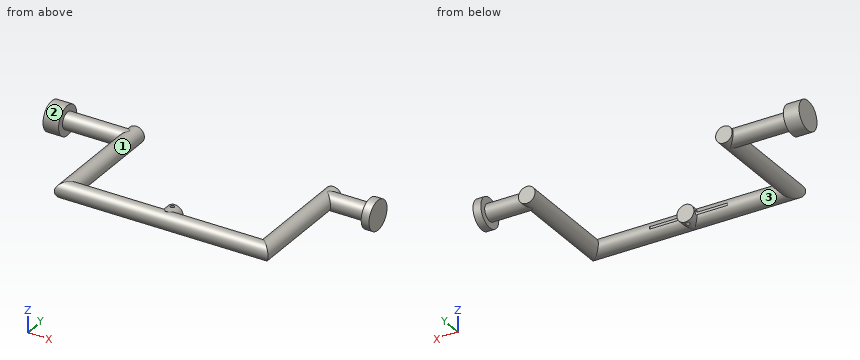
Autodesk Inventor part; units mm, degrees
ref_plane "Work Plane1" through (-126.3, 142.5, 0) normal (0, 1, 0) x (-1, 0, 0)
ref_plane "Work Plane2" through (0, 0, 0) normal (0, 1, 0) x (-1, 0, 0)
ref_plane "Work Plane3" through (0, 0, 0) normal (0, 0, 1) x (1, 0, 0)
sketch "Sketch1" plane through (0, 0, 0) normal (0, 0, 1) x (1, 0, 0)
  line L0 (-126.3, 0) -> (126.3, 0)
  line L1 (126.3, 0) -> (126.3, 142.5)
  line L2 (126.3, 0) -> (268.8, 0) construction
  line L3 (-126.3, 0) -> (-126.3, 142.5)
  point P0 (0, 0)
  dimension "d0" = 252.6
  dimension "d1" = 142.5
  dimension "d2" = 90
  dimension "d3" = 142.5
ref_plane "Work Plane1" through (-126.3, 142.5, 0) normal (0, 1, 0) x (-1, 0, 0)
sketch "Sketch2" plane through (-126.3, 142.5, 0) normal (0, 1, 0) x (-1, 0, 0)
  circle A0 centre (0, 0) radius 10.65
  point P0 (-126.3, 0)
  dimension "d4" = 21.3
sweep "Sweep1" add profiles "Sketch2" path "Sketch1"
ref_plane "Work Plane2" through (0, 0, 0) normal (0, 1, 0) x (-1, 0, 0)
sketch "Sketch3" plane through (0, 0, 0) normal (0, 1, 0) x (-1, 0, 0)
  circle A0 centre (0, 0) radius 11
  dimension "d8" = 22
extrude "Extrusion1" add sketch "Sketch3" along normal blind 17.5
ref_plane "Work Plane3" through (0, 0, 0) normal (0, 0, 1) x (1, 0, 0)
sketch "Sketch4" plane through (0, 0, 0) normal (0, 0, 1) x (1, 0, 0)
  circle A0 centre (0, 12.5) radius 2.5
  point P0 (0, 0)
  dimension "d12" = 5
extrude "Extrusion2" cut sketch "Sketch4" along normal mid plane 100
ref_plane "Work Plane4" through (0, 0, 0) normal (1, 0, 0) x (0, 1, 0)
sketch "Sketch5" plane through (0, 0, 0) normal (1, 0, 0) x (0, 1, 0)
  circle A0 centre (12.5, 0) radius 2.5
  point P0 (0, 0)
  dimension "d16" = 5
extrude "Extrusion3" cut sketch "Sketch5" along normal mid plane 100
sketch "Sketch6" plane through (-126.3, 142.5, 0) normal (0, 1, 0) x (1, 0, 0)
  circle A0 centre (0, 0) radius 10.65
  point P0 (126.3, 0)
sketch "Sketch7" plane through (126.3, 142.5, 0) normal (0, 1, 0) x (1, 0, 0)
  circle A0 centre (0, 0) radius 10.65
  point P0 (-126.3, 0)
ref_plane "Work Plane6" through (126.3, 0, 0) normal (1, 0, 0) x (0, 1, 0)
ref_plane "Work Plane7" through (-126.3, 0, 0) normal (1, 0, 0) x (0, 1, 0)
sketch "Sketch8" plane through (-126.3, 0, 0) normal (1, 0, 0) x (0, 1, 0)
  line L0 (142.5, -10.65) -> (142.5, 10.65)
  circle A0 centre (130, 0) radius 10.65
  point P0 (0, 0)
  point P1 (142.5, 0)
  dimension "d21" = 21.3
extrude "Extrusion4" add sketch "Sketch8" against normal blind 100
sketch "Sketch9" plane through (126.3, 0, 0) normal (1, 0, 0) x (0, 1, 0)
  circle A0 centre (130, 0) radius 10.65
  circle A1 centre (130, 0) radius 10.65
  point P0 (0, 0)
extrude "Extrusion5" add sketch "Sketch9" along normal blind 100
sketch "Sketch10" plane through (-226.3, 130, 0) normal (-1, 0, 0) x (0, 0, 1)
  circle A0 centre (0, 0) radius 18.7623
  point P0 (0, -130)
extrude "Extrusion6" add sketch "Sketch10" against normal blind 20
sketch "Sketch11" plane through (226.3, 130, 0) normal (1, 0, 0) x (0, 0, -1)
  circle A0 centre (0, 0) radius 10.65
  circle A1 centre (0, 0) radius 18.7623
  point P0 (0, -130)
extrude "Extrusion7" add sketch "Sketch11" against normal blind 45 contours A0 | A1
sketch "Sketch12" plane through (226.3, 130, 0) normal (1, 0, 0) x (0, 0, -1)
  circle A0 centre (0, 0) radius 18.7623
  point P0 (0, -130)
extrude "Extrusion8" cut sketch "Sketch12" against normal blind 35
properties part number "newhands" material "PVC-Piping"
Input: part model. Units: mm. Frame: model coordinates. Face numbers are marked on the shaded views. Round coordinates to 2 decimals unless told otherwise and drop trailing zeros. Loops run counter-clockwise (first coordinate to the right, second up) from the corner with the lowest first, then second, coordinate; pieces in that order, holes last.
1) Section query A-A on y = 60. Return the cut outline in (x, z), plus the area to 3 significant figures.
Ans:
outline: circle Ø21.3 at (-126.3, 0); circle Ø21.3 at (126.3, 0)
area: 713 mm2
2) Pull-direction query (X, two-part tool) for the marked faces 1, 2 and 3; classes: released by +X, released by -X, zero draft, split by the parting line, or undercut.
Ans:
face 1: undercut
face 2: zero draft
face 3: undercut
3) Material intervals for line 1 (X direction, y = 66, z = 0); line 2 (Y direction, x = 0, z = -2.5); line 3 (Y direction, x = 0, z = 4), sorted ascending.
Ans:
line 1: x = -136.95 to -115.65, 115.65 to 136.95
line 2: y = -10.35 to 10, 15 to 17.5
line 3: y = -9.87 to 10, 15 to 17.5
4) Section query C-C on x = 130. Return the cut outline in (y, z).
Ans:
outline: (-3.7, -9.99) - (126.3, -9.99) arc R10.65 ccw to (133.7, -9.99) - (142.5, -9.99) - (142.5, 9.99) - (133.7, 9.99) arc R10.65 ccw to (126.3, 9.99) - (-3.7, 9.99) arc R10.65 ccw to start
5) Section query B-B on x = -180. Return the cut outline in (y, z).
Ans:
outline: circle Ø21.3 at (130, 0)
6) Pin query (flat end, axial travel): pin 1 (6 mm diameter, centred on y = 12.5, z = 0, fed in from +X); pin 2 (5 mm diameter, centred on y = 59, z = -3, fed in from -X); pin 3 (6.5 mm diameter, centred on x = 128, z = 3, fed in from +Y). Return the tip coordinate at first contact, or that it passes through.
Ans:
pin 1: stops at x = 136.95
pin 2: stops at x = -136.94
pin 3: stops at y = 142.5
